Source: CAD feature listing. Evaluate the final solid. Frame: model axes, mm. A direction names the side the tool comes from. Give positions to 0.01 mm unless a question says otherwise; leave off trailing zeros. Write each loop counter-clockwise with the first axis right and the second up, starting at its lowest first coordinate (ties: lowest second). Pieces come first, ordered by that corner, then holes. Notation, with made-up numbers: M -38.5,12 L -30.5,12 A17 ccw -30.5,42 Z; hole C 23,47 d4. An arc over 180 degrees is marked long. Return JSON: item names as keys, results as strings.
```python
from build123d import *

# Parameters (mm, degrees)
F0_W     = 17.653
F0_H     = 1.651
F0_H_2   = 6.35
F0_R     = 1.905
F0_H_3   = 1.397
F0_H_4   = 1.143
F1_DEPTH = 3.175


with BuildPart() as f1:
    # F0 (on Top) → F1 (new body)
    with BuildSketch(Plane.XY):
        with Locations((0, -4.0005)):
            Rectangle(F0_W, F0_H)
        Rectangle(F0_W, F0_H_2)
        with Locations((-5.0165, 0)):
            Circle(F0_R, mode=Mode.SUBTRACT)
        with Locations((5.0165, 0)):
            Circle(F0_R, mode=Mode.SUBTRACT)
        Polygon((8.8265, 3.175), (8.8265, -3.175), (8.8265, -4.826), (12.0015, -4.826), (12.0015, 3.175), align=None)
        Polygon((-8.8265, -4.826), (-8.8265, -3.175), (-8.8265, 3.175), (-12.0015, 3.175), (-12.0015, -4.826), align=None)
        Polygon((15.1765, 3.175), (12.0015, 3.175), (12.0015, -4.826), (15.1765, -4.826), (15.1765, -4.572), (15.1765, -3.175), align=None)
        Polygon((-12.0015, -4.826), (-12.0015, 3.175), (-15.1765, 3.175), (-15.1765, -3.175), (-15.1765, -4.826), align=None)
        with Locations((24.003, 0)):
            Rectangle(F0_W, F0_H_2)
        with Locations((18.9865, 0)):
            Circle(F0_R, mode=Mode.SUBTRACT)
        with Locations((29.0195, 0)):
            Circle(F0_R, mode=Mode.SUBTRACT)
        with Locations((-24.003, 0)):
            Rectangle(F0_W, F0_H_2)
        with Locations((-29.0195, 0)):
            Circle(F0_R, mode=Mode.SUBTRACT)
        with Locations((-18.9865, 0)):
            Circle(F0_R, mode=Mode.SUBTRACT)
        Polygon((-15.1765, -5.08), (-15.1765, -4.826), (-15.1765, -3.175), (-32.8295, -3.175), (-32.8295, -5.08), align=None)
        with Locations((24.003, -3.8735)):
            Rectangle(F0_W, F0_H_3)
        Polygon((36.0045, 3.175), (32.8295, 3.175), (32.8295, -3.175), (32.8295, -4.572), (36.0045, -4.572), align=None)
        Polygon((39.1795, 3.175), (36.0045, 3.175), (36.0045, -4.572), (39.1795, -4.572), (39.1795, -4.318), (39.1795, -3.175), align=None)
        with Locations((48.006, 0)):
            Rectangle(F0_W, F0_H_2)
        with Locations((42.9895, 0)):
            Circle(F0_R, mode=Mode.SUBTRACT)
        with Locations((53.0225, 0)):
            Circle(F0_R, mode=Mode.SUBTRACT)
        with Locations((48.006, -3.7465)):
            Rectangle(F0_W, F0_H_4)
        Polygon((63.1825, 3.175), (56.8325, 3.175), (56.8325, -3.175), (56.8325, -4.318), (63.1825, -4.318), align=None)
    extrude(amount=F1_DEPTH)


solid = f1.part
```
1) Cut plane D-D, the plane x = 49.5. Return the cut outline in (y, z) (3 decimals).
Numbers:
{"outline": "M -4.318,0 L 3.175,0 L 3.175,3.175 L -4.318,3.175 Z"}
2) Set-up query: faces 4 (the face through (16, 3.175, 2)), 5 (the face through (51, -4.318, 2)). Return all of +Z, -Z, +X, -X, +Y, -Y with unobstructed straight access to the full face (end or side cutting, diameter ignored); none if empty.
Numbers:
{"face 4": "+Z, -Z, +X, -X, +Y", "face 5": "+Z, -Z, +X, -Y"}
3) Cut plane C-C, the plane x = 25. Return the cut outline in (y, z) (3 decimals).
Numbers:
{"outline": "M -4.572,0 L 3.175,0 L 3.175,3.175 L -4.572,3.175 Z"}
4) Cut plane A-A, the plane z = 0.8. Give the number of separate pieces and of enclosed holes in the cut face, then the cut area to 3 significant figures.
Numbers:
{"separate pieces": "1", "enclosed holes": "8", "area": "663 mm²"}
5) Line query: line 1 (Y direction, x = 48.5, z = 2.3) (3 decimals); line 2 (Y direction, x = -8, z = 1.35) (3 decimals); line 3 (Y direction, x = -20, z = 2.25) (3 decimals). Output: solid intervals per line, ascending. Write a range as [from, to].
Numbers:
{"line 1": "y = [-4.318, 3.175]", "line 2": "y = [-4.826, 3.175]", "line 3": "y = [-5.08, -1.613], [1.613, 3.175]"}
6) Contact query for flat-ended pins moving along their axis: pin 1 Ø1 at (x, z) = (5.5, 2) entering from -Y; pin 2 Ø3.5 at (x, y) = (-18.99, 0) entering from +Z; pin 3 Ø1.6 at (x, z) = (25, 1.5) entering from -Y; pin 4 Ø1.6 at (x, z) = (52.5, 2) entering from -Y. Output: stop coordinate, or through.
Numbers:
{"pin 1": "stops at y = -4.83", "pin 2": "passes through", "pin 3": "stops at y = -4.57", "pin 4": "stops at y = -4.32"}
7) Draft query along X for faces 1 (the face through (-27.26, -0.73, 1.57)), 2 (the face through (15, -1, 0)), 3 (the face through (-32.829, -1, 2)). Return one class per face: released by +X, released by -X, zero draft, split by the parting line, or undercut.
Numbers:
{"face 1": "undercut", "face 2": "zero draft", "face 3": "released by -X"}
